Build history of the part. All positions in model axes, mm. A direction names the side the tool comes from. Round coordinates to 2 decimals unless told otherwise and drop trailing zeros. Loops run counter-clockwise (first coordinate to the right, second up) from the corner with the lowest first, then second, coordinate; pieces in that order, holes last. Notation, with made-up numbers: (2.25, 56) - (21.25, 56) arc R24 ccw to (21.25, 67) - close; hole circle Ø8 at (-11.5, 1.5). An arc over 180 degrees is marked (long way). Use one line per item in the form item = value. Start each with the question number.
Q1. Pin check, flat tips, straight feed: pin 1 (4 mm diameter, centred on x = -52.4, y = -11.43, fed in from +Z); pin 2 (7 mm diameter, centred on x = -60, y = -30.5, fed in from +Z); pin 3 (3 mm diameter, centred on x = -36.1, y = -39.67, fed in from -Z). Stop position of each tip, or through.
Q2. Saw through at B-B (z = -2.4). Give the cut face in (x, y), then the cut area to 3 significant figures.
Q3. Saw through at C-C (x = -47). Give the cut face in (y, z).
Q4. 3-axis set-ups, long thin cutter, end or side, ignore diameter. For faces 4 (the face through (-70.174, -22.082, -1.479)), 5 (the face through (-51.1, -29.69, -0.79)): which of +Z, -Z, +X, -X, +Y, -Y reach the whole face in a straight line?
Q5. Mould opens along Y. For faces 1 (the face through (-57, -33, -1.6)), 2 (the face through (-49, -31, 0)), 3 (the face through (-40.918, -23.328, -1.479)) say: released by +Y, released by -Y, zero draft, split by the parting line, or undercut.
Q6. Drill centre lines: line 1 (Y direction, x = -51.5, z = -1.4); line 2 (X direction, y = -22, z = -2.6); line 3 (Y direction, x = -61, z = -2.8). Where is each one in solid material? Low to high.
Q7. Saw through at A-A (x = -37). Give the cut face in (y, z), then the cut area to 3 significant figures.
Q8. Saw through at D-D (y = -45.5). Give the cut face in (x, z).
```python
from build123d import *

# Parameters (mm, degrees)
SKETCH2_R           = 1.6
BOSS_EXTRUDE1_DEPTH = 3
FILLET1_R           = 2
CUT_EXTRUDE1_DEPTH  = 1.6


with BuildPart() as part:
    # Sketch2 → Boss-Extrude1 (new body)
    with BuildSketch(Plane.XY):
        Polygon((-77.786584036, -21.469684303), (-50.939796518, -5.969684303), (-30.639796518, -41.130315697), (-57.486584036, -56.630315697), (-61.986584036, -48.836087063), (-57.656457017, -46.336087063), (-68.956457017, -26.763912937), (-73.286584036, -29.263912937), align=None)
        with Locations((-52.403898133, -11.433785918)):
            Circle(SKETCH2_R, mode=Mode.SUBTRACT)
        with Locations((-36.103898133, -39.666214082)):
            Circle(SKETCH2_R, mode=Mode.SUBTRACT)
        with Locations((-55.390275833, -50.812719363)):
            Circle(SKETCH2_R, mode=Mode.SUBTRACT)
        with Locations((-71.70024372, -22.563026312)):
            Circle(SKETCH2_R, mode=Mode.SUBTRACT)
    extrude(amount=-BOSS_EXTRUDE1_DEPTH)

    # Fillet1
    fillet1_edges = [part.edges().sort_by_distance(p)[0] for p in [
        (-77.786584036, -21.469684303, -1.5),
        (-50.939796518, -5.969684303, -1.5),
        (-30.639796518, -41.130315697, -1.5),
        (-57.486584036, -56.630315697, -1.5),
        (-61.986584036, -48.836087063, -1.5),
        (-73.286584036, -29.263912937, -1.5),
    ]]
    fillet(fillet1_edges, radius=FILLET1_R)

    # Sketch3 → Cut-Extrude1 (cut)
    with BuildSketch(Plane.XY):
        Polygon((-68.956457017, -26.763912937), (-57.656457017, -46.336087063), (-45.532101364, -39.336087063), (-56.832101364, -19.763912937), align=None)
    extrude(amount=-CUT_EXTRUDE1_DEPTH, mode=Mode.SUBTRACT)


solid = part.part
```
Report:
q1.pin_1 = 0
q1.pin_2 = -1.6
q1.pin_3 = through
q2.outline = (-76.79, -23.2) - (-74.29, -27.53) arc R2 ccw to (-71.55, -28.26) - (-68.96, -26.76) - (-57.66, -46.34) - (-60.25, -47.84) arc R2 ccw to (-60.99, -50.57) - (-58.49, -54.9) arc R2 ccw to (-55.75, -55.63) - (-32.37, -42.13) arc R2 ccw to (-31.64, -39.4) - (-49.94, -7.7) arc R2 ccw to (-52.67, -6.97) - (-76.05, -20.47) arc R2 ccw to start; hole circle Ø3.2 at (-71.7, -22.56); hole circle Ø3.2 at (-55.39, -50.81); hole circle Ø3.2 at (-52.4, -11.43); hole circle Ø3.2 at (-36.1, -39.67)
q2.area = 1,110 mm²
q3.outline = (-50.58, -3) - (-12.79, -3) - (-12.79, 0) - (-36.79, 0) - (-36.79, -1.6) - (-40.18, -1.6) - (-40.18, 0) - (-50.58, 0) - close
q4.face_4 = +Z, -Z
q4.face_5 = +Z
q5.face_1 = undercut
q5.face_2 = zero draft
q5.face_3 = released by +Y
q6.line_1 = -53.17 to -42.78, -29 to -12.75, -10.11 to -6.71
q6.line_2 = -77.04 to -73.2, -70.2 to -41.68
q6.line_3 = -50.54 to -48.59, -40.54 to -11.78
q7.outline = (-44.8, -3) - (-40.99, -3) - (-40.99, 0) - (-44.8, 0) - close; (-38.34, -3) - (-30.11, -3) - (-30.11, 0) - (-38.34, 0) - close
q7.area = 36.1 mm²
q8.outline = (-58.14, -3) - (-38.21, -3) - (-38.21, 0) - (-56.21, 0) - (-56.21, -1.6) - (-58.14, -1.6) - close
